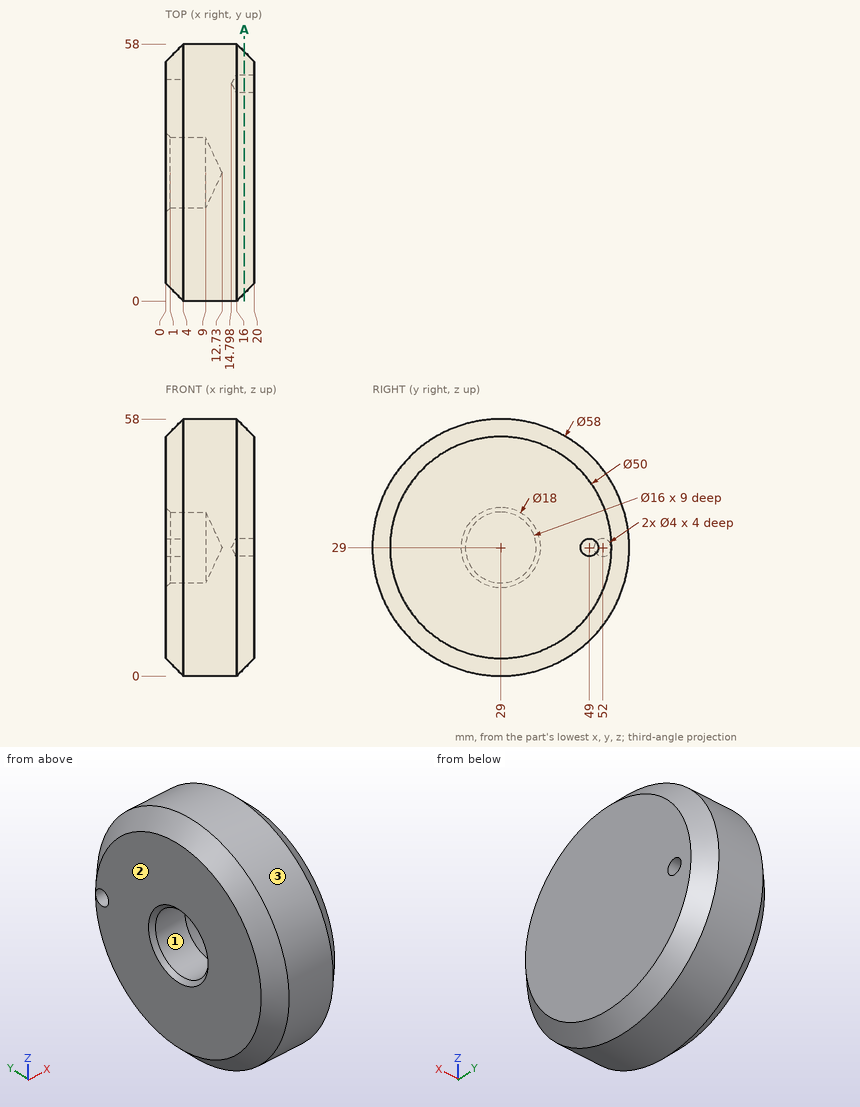
Answer from the drawing. Dimensions are ordinates in mm from the lowest x, y and z of the part. Coordinates: 2 decimals unless noted, no trailing zeros. Write each loop counter-clockwise with the first axis right and the second up, starting at its lowest first coordinate (ties: lowest second). Pieces come first, ordered by that corner, then holes. Notation, with made-up numbers: (74.25, 46.5) - (83.25, 46.5) arc R11 cw to (83.25, 60.5) - close; hole circle Ø11 at (-16.5, -15.75). An arc over 180 degrees is marked (long way). One line per question, with ' | ' between items.
Q1. Each of these flat-tipped pins is pushed along its axis until it touches: P1, Ø4, axis at x = 3.5, z = 51.5, coming from the -Y side; P2, Ø1, axis at x = 16, y = 22.5, coming from the +Z side; P3, Ø6, axis at x = 14.5, y = 33, coming from the +Z side. Where does it stop, or does it pass through?
Result set:
P1: y = 8.55 | P2: z = 57.37 | P3: z = 57.98
Q2. Consider L1, parallel to Y at x = 3, z = 29; L2, parallel to Z at x = 17.5, y = 49 (1 decimal); L3, parallel to Y at x = 3.5, z = 29. Determine where each line is inside the solid, lowest interval first. Write a range as [from, to].
Result set:
L1: [1, 21], [37, 50], [54, 57] | L2: [10.1, 27], [31, 47.9] | L3: [0.5, 21], [37, 50], [54, 57.5]
Q3. Determine the mould class of the marked faces 1, 2 and 3 for opening direction Y: +Y half, -Y half, draft (parallel to the pull), parting line (faces both ways), or undercut.
Result set:
face 1: undercut | face 2: draft | face 3: parting line
Q4. Find section A-A, the plane x = 17.75. Write down the section's boundary in (y, z), plus the area to 3 significant figures.
Result set:
outline: circle Ø54.5 at (29, 29); hole circle Ø4 at (49, 29) | area: 2,320 mm^2
